For this review, use the dimensioned drawing (mm, ordinates from the lowest corner) and the shaded views. A direction names the side the tool comes from. Coordinates: 2 decimals unless noted, no trailing zeros. Loops run counter-clockwise (first coordinate to the right, second up) from the corner with the lowest first, then second, coordinate; pieces in that order, holes last.
1. Machinability: for the marked faces 5 and 6, which of the approach directions +Z, -Z, +X, -X, +Y, -Y give a long, thin tool a straight path to every point of the face, cutting with its end or side? Answer none if there is none.
2. Take a section at B-B, the plane x = 43.5. State the section outline as (y, z) points, then the cut area to 3 significant figures.
3. To check wall thickness, follow probe 1 along Z at (x, y) = (20, 8.5); probe 2 along Y at (x, z) = (58, 4.5); probe 3 along Y at (x, z) = (8, 1) (1 decimal). State the ranges of each line that lie inside material, in increasing order.
4. Mouldability with a two-part tool opening along Y and no side actions: class the marked faces 1, 2, 3 and 4 as pulls with the +Y half, pulls with the -Y half, needs draft (parallel to the pull), parting line crosses it, or undercut.
5. Take a section at A-A, the plane y = 20. State the section outline as (x, z) points, then the cut area to 3 significant figures.
6. Clearance check with a flat-ended pin moving along its axis: P1, Ø6.5, axis at x = 6.81, y = 83.18, coming from the -Z side. State where the tip first meets the part, or that it passes through.
7. Take a section at C-C, the plane x = 70. State the section outline as (y, z) points.
8. Take a section at D-D, the plane x = 83.89. State the section outline as (y, z) points.
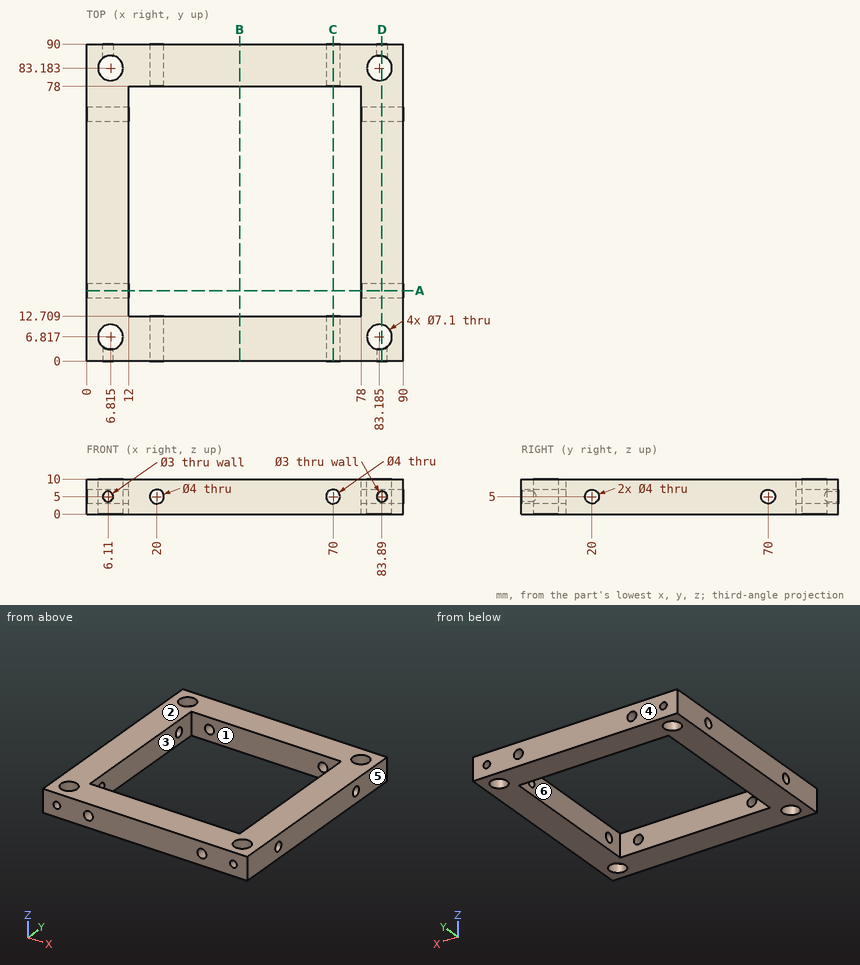
Results list:
1. face 5: +Z, -Z, +X, +Y, -Y
1. face 6: +Z, -Z
2. outline: (0, 0) - (12.71, 0) - (12.71, 10) - (0, 10) - close; (78, 0) - (90, 0) - (90, 10) - (78, 10) - close
2. area: 247 mm2
3. probe 1: z = 0 to 3, 7 to 10
3. probe 2: y = 0 to 12.71, 78 to 90
3. probe 3: y = 0 to 3.5, 10.2 to 79.8, 86.5 to 90
4. face 1: undercut
4. face 2: needs draft
4. face 3: undercut
4. face 4: pulls with the +Y half
5. outline: (0, 0) - (12, 0) - (12, 3) - (0, 3) - close; (0, 7) - (12, 7) - (12, 10) - (0, 10) - close; (78, 0) - (90, 0) - (90, 3) - (78, 3) - close; (78, 7) - (90, 7) - (90, 10) - (78, 10) - close
5. area: 144 mm2
6. P1: passes through
7. outline: (0, 0) - (12.71, 0) - (12.71, 3) - (0, 3) - close; (0, 7) - (12.71, 7) - (12.71, 10) - (0, 10) - close; (78, 0) - (90, 0) - (90, 3) - (78, 3) - close; (78, 7) - (90, 7) - (90, 10) - (78, 10) - close
8. outline: (0, 0) - (3.34, 0) - (3.34, 3.5) - (0, 3.5) - close; (0, 6.5) - (3.34, 6.5) - (3.34, 10) - (0, 10) - close; (10.3, 0) - (79.7, 0) - (79.7, 10) - (10.3, 10) - close; (86.66, 0) - (90, 0) - (90, 3.5) - (86.66, 3.5) - close; (86.66, 6.5) - (90, 6.5) - (90, 10) - (86.66, 10) - close; hole circle Ø4 at (20, 5); hole circle Ø4 at (70, 5)
